from build123d import *

# Parameters (mm, degrees)
SKETCH1_W           = 60
SKETCH1_H           = 60
SKETCH1_W_2         = 50
SKETCH1_H_2         = 50
BOSS_EXTRUDE1_DEPTH = 60
SKETCH2_W           = 60
SKETCH2_H           = 60
BOSS_EXTRUDE2_DEPTH = 5
SKETCH3_R           = 1.25
CUT_EXTRUDE1_DEPTH  = 5
CUT_EXTRUDE2_REACH  = 62
SKETCH4_R           = 1.25


with BuildPart() as part:
    # Sketch1 → Boss-Extrude1 (new body)
    with BuildSketch(Plane(origin=(0, 0, 0), x_dir=(1, 0, 0), z_dir=(0, 1, 0))):
        Rectangle(SKETCH1_W, SKETCH1_H)
        Rectangle(SKETCH1_W_2, SKETCH1_H_2, mode=Mode.SUBTRACT)
    extrude(amount=BOSS_EXTRUDE1_DEPTH)

    # Sketch2 → Boss-Extrude2 (add)
    with BuildSketch(Plane.XZ):
        Rectangle(SKETCH2_W, SKETCH2_H)
    extrude(amount=BOSS_EXTRUDE2_DEPTH)

    # Sketch3 → Cut-Extrude1 (cut)
    with BuildSketch(Plane(origin=(0, 0, -30), x_dir=(-1, 0, 0), z_dir=(0, 0, -1))):
        with Locations((0, 2.5)):
            Circle(SKETCH3_R)
        with Locations((0, 8.1)):
            Circle(SKETCH3_R)
    extrude(amount=-CUT_EXTRUDE1_DEPTH, mode=Mode.SUBTRACT)

    # Sketch4 → Cut-Extrude2 (cut, up to next)
    with BuildSketch(Plane(origin=(0, 0, -30), x_dir=(-1, 0, 0), z_dir=(0, 0, -1)), mode=Mode.PRIVATE) as cut_extrude2_sk1:
        with Locations((-13.176528006, 8.1)):
            Circle(SKETCH4_R)
    cut_extrude2_tool1 = extrude(cut_extrude2_sk1.sketch, amount=-CUT_EXTRUDE2_REACH, mode=Mode.PRIVATE) & part.part
    add(cut_extrude2_tool1.solids().sort_by_distance((13.176528, 8.1, -30))[0], mode=Mode.SUBTRACT)


solid = part.part
Source: CAD feature listing. Evaluate the final solid. Frame: model axes, mm. A direction names the side the tool comes from. Coordinates: 2 decimals unless noted, no trailing zeros. Order: outer loops, then holes, each group sorted by start corner. A loop starts at its lowest first (then second) coordinate and runs counter-clockwise, first axis right, second up. Notation, with made-up numbers: M 43,69.5 L 96,69.5 A13 ccw 96,86.5 Z; hole C 17.25,1.25 d7. An arc over 180 degrees is marked long. Write each question's results on one line, items separated by ' | '. Start each with the question number.
1. Section C-C, the plane z = 4.5. Return the cut outline in (x, y).
2. Draft query along X for faces 4 (the face through (0, 28, -30)), 5 (the face through (30, 28, 0)), 6 (the face through (25, 30, 0)). Return one class per face: +X half, -X half, draft (parallel to the pull), parting line (faces both ways), or undercut.
3. Section B-B, the plane x = 0. Return the cut outline in (y, z), then the cut area to 3 significant figures.
4. Section D-D, the plane x = 19.5. Return the cut outline in (y, z).
5. Material intervals for L1, parallel to Z at x = -15, y = 13.5; L2, parallel to Y at x = 0, z = -28, sorted ascending.
6. Section A-A, the plane y = 8.1. Return the cut outline in (x, z), then the cut area to 4 significant figures.
7. Reachability of faces 1 (the face through (12.022, 7.621, -27.535)), 2 (the face through (-30, 28, 0)), 3 (the face through (0, 0, 0)) from +Z, -Z, +X, -X, +Y, -Y: full face, straight path, thin tool, end or side. Return the list, or none.
8. Pin query (flat end, axial travel): pin 1 (12 mm diameter, centred on x = -14, z = -4.5, fed in from +Y). Return the tip coordinate at first contact, or that it passes through.
Solution:
1) outline: M -30,-5 L 30,-5 L 30,60 L 25,60 L 25,0 L -25,0 L -25,60 L -30,60 Z
2) face 4: draft | face 5: +X half | face 6: undercut
3) outline: M -5,-30 L 1.25,-30 L 1.25,-25 L 0,-25 L 0,25 L 60,25 L 60,30 L -5,30 Z; M 3.75,-30 L 6.85,-30 L 6.85,-25 L 3.75,-25 Z; M 9.35,-30 L 60,-30 L 60,-25 L 9.35,-25 Z | area: 875 mm²
4) outline: M -5,-30 L 60,-30 L 60,-25 L 0,-25 L 0,25 L 60,25 L 60,30 L -5,30 Z
5) L1: -30 to -25, 25 to 30 | L2: -5 to 1.25, 3.75 to 6.85, 9.35 to 60
6) outline: M -30,-30 L -1.25,-30 L -1.25,-25 L -25,-25 L -25,25 L 25,25 L 25,-25 L 14.43,-25 L 14.43,-30 L 30,-30 L 30,30 L -30,30 Z; M 1.25,-30 L 11.93,-30 L 11.93,-25 L 1.25,-25 Z | area: 1,075 mm²
7) face 1: -Z | face 2: +Z, -Z, -X, +Y, -Y | face 3: +Y
8) pin 1: y = 0
